Can you work these out from the model? Positions are in its coordinate system, mm. A direction names the side the tool comes from. Give positions to 0.01 mm unless a question says otherwise; leave off trailing zeros. Write each loop counter-clockwise with the first axis right and the second up, starting at its lowest first coordinate (ties: lowest second). Pieces come first, ordered by that corner, then holes. Notation, with made-up numbers: M -15,19.5 L 18,19.5 A14 ccw 18,43.5 Z; hole C -18.5,24 d8. An arc over 180 degrees is marked long. Write each question's results on one line, items separated by ' | '.
from build123d import *

# Parameters (mm, degrees)
SKETCH1_R           = 27.5
SKETCH1_R_2         = 22.5
BOSS_EXTRUDE1_DEPTH = 130
CUT_EXTRUDE1_START  = -7
CUT_EXTRUDE1_DEPTH  = 7


with BuildPart() as part:
    # Sketch1 → Boss-Extrude1 (new body)
    with BuildSketch(Plane(origin=(0, 0, 0), x_dir=(1, 0, 0), z_dir=(0, 1, 0))):
        with Locations(Location((0, 0, 0), (0, 0, 270))):
            Circle(SKETCH1_R)
        with Locations(Location((0, 0, 0), (0, 0, 270))):
            Circle(SKETCH1_R_2, mode=Mode.SUBTRACT)
    extrude(amount=BOSS_EXTRUDE1_DEPTH)

    # Sketch2 → Cut-Extrude1 (cut)
    with BuildSketch(Plane(origin=(0, 130, 0), x_dir=(1, 0, 0), z_dir=(0, 1, 0)).offset(CUT_EXTRUDE1_START)):
        with BuildLine():
            Line((-27.407799985, 2.25), (-22.387217335, 2.25))
            ThreePointArc((-22.387217335, 2.25), (-22.5, 0), (-22.387217335, -2.25))
            Line((-22.387217335, -2.25), (-27.407799985, -2.25))
            ThreePointArc((-27.407799985, -2.25), (-27.5, 0), (-27.407799985, 2.25))
        make_face()
        with BuildLine():
            Line((27.407799985, -2.25), (22.387217335, -2.25))
            ThreePointArc((22.387217335, -2.25), (22.5, 0), (22.387217335, 2.25))
            Line((22.387217335, 2.25), (27.407799985, 2.25))
            ThreePointArc((27.407799985, 2.25), (27.5, 0), (27.407799985, -2.25))
        make_face()
        with BuildLine():
            Line((-2.25, 27.407799985), (-2.25, 22.387217335))
            ThreePointArc((-2.25, 22.387217335), (0, 22.5), (2.25, 22.387217335))
            Line((2.25, 22.387217335), (2.25, 27.407799985))
            ThreePointArc((2.25, 27.407799985), (0, 27.5), (-2.25, 27.407799985))
        make_face()
        with BuildLine():
            Line((-2.25, -27.407799985), (-2.25, -22.387217335))
            ThreePointArc((-2.25, -22.387217335), (0, -22.5), (2.25, -22.387217335))
            Line((2.25, -22.387217335), (2.25, -27.407799985))
            ThreePointArc((2.25, -27.407799985), (0, -27.5), (-2.25, -27.407799985))
        make_face()
    extrude(amount=CUT_EXTRUDE1_DEPTH, mode=Mode.SUBTRACT)


solid = part.part
Item 1: If I drill on line 1 (X direction, y = 68, z = 0); line 2 (X direction, y = 121, z = 5); line 3 (Z direction, x = -3.5, y = 98.5), over which ranges is the centre line in solid material (lowest first)? Write a range as from..to.
Geometry says:
line 1: x = -27.5..-22.5, 22.5..27.5 | line 2: x = -27.04..-21.94, 21.94..27.04 | line 3: z = -27.28..-22.23, 22.23..27.28
Item 2: I want a section at B-B, the plane x = 0. Please give me the cut outline in (y, z).
Geometry says:
outline: M 0,-27.5 L 123,-27.5 L 123,-22.5 L 0,-22.5 Z; M 0,22.5 L 123,22.5 L 123,27.5 L 0,27.5 Z
Item 3: I'm going to push flat-ended pins straight in: pin 1 (2.5 mm diameter, centred on y = 127, z = -25, fed in from -X); pin 2 (2.5 mm diameter, centred on x = 25.5, z = 0, fed in from +Y); pin 3 (1.5 mm diameter, centred on y = 125.5, z = 23.5, fed in from -X). Where does each tip first touch, or does it pass through?
Geometry says:
pin 1: stops at x = -13.86 | pin 2: stops at y = 123 | pin 3: stops at x = -15.45
Item 4: I want a section at C-C, the plane y = 21. Please give me the cut outline in (x, z).
Geometry says:
outline: C 0,0 d55; hole C 0,0 d45
Item 5: For faces 4 (the face through (0, 0, -23)), 5 (the face through (25, 123, 0)), 6 (the face through (2.25, 126, -25)), which set-ups out of +Z, -Z, +X, -X, +Y, -Y let a thin tool reach every point of the face, with its end or its side?
Geometry says:
face 4: +Z, -Z, +X, -X, -Y | face 5: +X, -X, +Y | face 6: +Z, -Z, +Y
Item 6: I want a section at A-A, the plane z = 0. Please give me the cut outline in (x, y).
Geometry says:
outline: M -27.5,0 L -22.5,0 L -22.5,123 L -27.5,123 Z; M 22.5,0 L 27.5,0 L 27.5,123 L 22.5,123 Z
Item 7: Thinking about a two-plate mould opening in Z: for faces 1 (the face through (-2.25, 126, 25)), 2 (the face through (8.26, 64.09, 26.23)), 3 (the face through (25, 126, 2.25)), which applies, +Z half, -Z half, draft (parallel to the pull), parting line (faces both ways), or undercut?
Geometry says:
face 1: draft | face 2: parting line | face 3: undercut
